Part model, mm, in its own coordinate system. Round coordinates to 2 decimals unless told otherwise and drop trailing zeros. Write each loop counter-clockwise with the first axis right and the second up, starting at its lowest first coordinate (ties: lowest second). Pieces come first, ordered by that corner, then holes. Notation, with made-up numbers: (-18.5, -21.5) -> (-9.5, -21.5) arc R20 cw to (-9.5, 8.5) -> close; hole circle Ø8 at (74.5, -19). An arc over 180 degrees is marked (long way). Use CSV: the item, a comma, the result in double quotes. Start each with the question number.
(1) Probe line 1 (Y direction, x = 1003.45, z = 89.5); line 2 (Z direction, x = 1005.1, y = 253); line 3 (Z direction, x = 1005.75, y = 304). List the from-to ranges inside material, lowest first. Write a range as [from, to].
(2) Saw through at B-B (z = 112). Give the cut face in (x, y).
(3) Saw through at C-C (y = 312.5). Give the cut face in (x, z).
(4) Drop flat-ended pins along their axis: pin 1 (3 mm diameter, centred on x = 1004, z = 119, fed in from +Y); pin 2 (3 mm diameter, centred on x = 1002.5, y = 319.5, fed in from -Z). Give the stop position or say it passes through.
(5) Saw through at A-A (x = 1000.9). Count the separate pieces of the cut face and the enclosed holes in it, plus the area to 3 significant figures.
```python
from build123d import *

# Parameters (mm, degrees)
PAD005_DEPTH             = 6
SKETCH025_R              = 2.1
HOLE006_DEPTH            = 25
SKETCH026_R              = 3.6
HOLE007_DEPTH            = 25
SKETCH027_R              = 2.65
HOLE008_DEPTH            = 25
SKETCH028_R              = 1.6
HOLE009_DEPTH            = 25
SKETCH029_R              = 12.5
POCKET001_DEPTH          = 6.001
SKETCH030_R              = 2.65
HOLE010_DEPTH            = 25
SKETCH031_R              = 2.65
HOLE011_DEPTH            = 25
SKETCH032_R              = 2.1
HOLE012_DEPTH            = 25
SKETCH033_R              = 4.21
POCKET_DEPTH             = 6.001
BODY013_ROLL_ANGLE       = 90
BODY013_PLACEMENT_ANGLE  = -90
CLONE005_PLACEMENT_ANGLE = 180
BODY014_PLACEMENT_ANGLE  = 180


with BuildPart() as part:
    # Sketch → Pad005 (new body)
    with BuildSketch(Plane.XY):
        with BuildLine():
            Line((-53.583397, -36.74454), (-53.583397, 3.25546))
            Line((-53.583397, 3.25546), (-13.583397, 3.25546))
            ThreePointArc((-13.583397, 3.25546), (-11.462077, 4.134139), (-10.583397, 6.25546))
            Line((-10.583397, 6.25546), (-10.583397, 27.066205))
            ThreePointArc((-7.583397, 30.066205), (-9.704717, 29.187525), (-10.583397, 27.066205))
            Line((-7.583397, 30.066205), (70.056603, 30.066205))
            Line((70.056603, 30.066205), (70.056603, -97.580221))
            ThreePointArc((67.056603, -100.580221), (69.177923, -99.701542), (70.056603, -97.580221))
            Line((67.056603, -100.580221), (-7.583397, -100.580221))
            ThreePointArc((-10.583397, -97.580221), (-9.704717, -99.701542), (-7.583397, -100.580221))
            Line((-10.583397, -97.580221), (-10.583397, -39.74454))
            ThreePointArc((-10.583397, -39.74454), (-11.462077, -37.62322), (-13.583397, -36.74454))
            Line((-13.583397, -36.74454), (-53.583397, -36.74454))
        make_face()
    extrude(amount=PAD005_DEPTH)

    # Sketch025 (on Face15 of Pad005) → Hole006 (cut)
    with BuildSketch(Plane.XY.offset(6)):
        with Locations((-43.583397, -6.74454)):
            Circle(SKETCH025_R)
        with Locations((-43.583397, -26.74454)):
            Circle(SKETCH025_R)
    extrude(amount=-HOLE006_DEPTH, mode=Mode.SUBTRACT)

    # Sketch026 (on Face5 of Hole006) → Hole007 (cut)
    with BuildSketch(Plane.XY.offset(6)):
        with Locations((-0.583397, -31.89454)):
            Circle(SKETCH026_R)
        with Locations((60.056603, -31.89454)):
            Circle(SKETCH026_R)
    extrude(amount=-HOLE007_DEPTH, mode=Mode.SUBTRACT)

    # Sketch027 (on Face5 of Hole007) → Hole008 (cut)
    with BuildSketch(Plane.XY.offset(6)):
        with Locations((-0.583397, -91.89454)):
            Circle(SKETCH027_R)
        with Locations((60.056603, -91.89454)):
            Circle(SKETCH027_R)
    extrude(amount=-HOLE008_DEPTH, mode=Mode.SUBTRACT)

    # Sketch028 (on Face5 of Hole008) → Hole009 (cut)
    with BuildSketch(Plane.XY.offset(6)):
        with Locations((14.236603, -0.39454)):
            Circle(SKETCH028_R)
        with Locations((45.236603, -0.39454)):
            Circle(SKETCH028_R)
        with Locations((14.236603, -31.39454)):
            Circle(SKETCH028_R)
        with Locations((45.236603, -31.39454)):
            Circle(SKETCH028_R)
    extrude(amount=-HOLE009_DEPTH, mode=Mode.SUBTRACT)

    # Sketch029 (on Face5 of Hole009) → Pocket001 (cut, through all)
    with BuildSketch(Plane.XY.offset(6)):
        with Locations((29.736603, -15.89454)):
            Circle(SKETCH029_R)
    extrude(amount=-POCKET001_DEPTH, mode=Mode.SUBTRACT)

    # Sketch030 (on Face4 of Clone004) → Hole010 (cut)
    with BuildSketch(Plane(origin=(0, 0, 0), x_dir=(1, 0, 0), z_dir=(0, 0, -1))):
        with Locations((40.056603, -20.10546)):
            Circle(SKETCH030_R)
        with Locations((60.056603, -20.10546)):
            Circle(SKETCH030_R)
    extrude(amount=-HOLE010_DEPTH, mode=Mode.SUBTRACT)

    # Sketch031 (on Face5 of Hole010) → Hole011 (cut)
    with BuildSketch(Plane.XY.offset(6)):
        with Locations((-23.583397, -6.74454)):
            Circle(SKETCH031_R)
        with Locations((-23.583397, -26.74454)):
            Circle(SKETCH031_R)
    extrude(amount=-HOLE011_DEPTH, mode=Mode.SUBTRACT)

    # Sketch032 (on Face5 of Hole011) → Hole012 (cut)
    with BuildSketch(Plane.XY.offset(6)):
        with Locations((29.736603, -75.580221)):
            Circle(SKETCH032_R)
    extrude(amount=-HOLE012_DEPTH, mode=Mode.SUBTRACT)

    # Sketch033 (on Face5 of Hole012) → Pocket (cut, through all)
    with BuildSketch(Plane.XY.offset(6)):
        with Locations((-23.583397, -16.74454)):
            Circle(SKETCH033_R)
    extrude(amount=-POCKET_DEPTH, mode=Mode.SUBTRACT)


with BuildPart() as part_1:
    # Body013 roll: moved
    add(part.part.rotate(Axis((0, 0, 0), (1, 0, 0)), BODY013_ROLL_ANGLE))


with BuildPart() as part_2:
    # Body013 placement: moved
    add(part_1.part.moved(Location((0, 283, 181.7))).rotate(Axis((0, 283, 181.7), (0, 0, 1)), BODY013_PLACEMENT_ANGLE))


with BuildPart() as part_3:
    # Clone005 placement: moved
    add(part_2.part.moved(Location((-6, 586.6, 0))).rotate(Axis((-6, 586.6, 0), (0, 0, 1)), CLONE005_PLACEMENT_ANGLE))


with BuildPart() as part_4:
    # Body014 placement: moved
    add(part_3.part.moved(Location((1000, 586.4, 0))).rotate(Axis((1000, 586.4, 0), (0, 0, 1)), BODY014_PLACEMENT_ANGLE))


solid = part_4.part
```
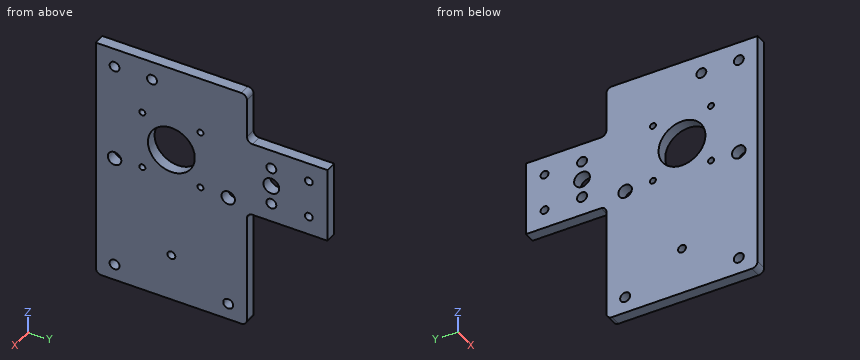
Answers:
1,line 1,"y = [212.74, 220.11], [225.38, 280.75], [286.02, 293.38]"
1,line 2,"z = [81.12, 104.02], [108.22, 153.31], [178.31, 211.77]"
1,line 3,"z = [144.96, 153.8], [156.11, 161.49], [168.43, 173.8], [176.11, 184.96]"
2,outline,"(1000, 212.74) -> (1006, 212.74) -> (1006, 293.38) -> (1000, 293.38) -> close"
3,outline,"(1000, 144.96) -> (1006, 144.96) -> (1006, 184.96) -> (1000, 184.96) -> close"
4,pin 1,"stops at y = 293.38"
4,pin 2,"stops at z = 144.96"
5,separate pieces,"1"
5,enclosed holes,"17"
5,area,"11,400 mm²"
